For this review, take the finished solid that the model builds, in its own axes (mm). A direction names the side the tool comes from. Round coordinates to 2 decimals unless told otherwise and drop trailing zeros. Loops run counter-clockwise (first coordinate to the right, second up) from the corner with the lowest first, then second, coordinate; pieces in that order, holes last.
1. Consider section A-A on x = -49. State the section outline as (y, z) points (3 decimals).
2. Clearance check with flat-ended pins moving along their axes: pin 1 Ø3 at (y, z) = (-0.5, -6) entering from +X; pin 2 Ø8 at (x, z) = (-28, -1.5) entering from +Y (3 decimals); pin 3 Ø8 at (x, z) = (-22.5, 0.5) entering from -Y (3 decimals). State where each tip first meets the part, or that it passes through.
3. Draft analysis for pull direction X (two halves, no side actions). For faces 1 (the cylindrical face through (-14.31, 2.33, -0.52)), 2 (the cylindrical face through (-8, 3.1, -0.69)), 3 (the conical face through (-58.165, -1.259, 3.996)), 4 (the flat face through (-63.5, 0, 0)), state which applies: released by +X, released by -X, zero draft, split by the parting line, or undercut.
4. To check wall thickness, follow line 1 along X through (y, z) = (-5.75, -7.25); line 2 along Y through (x, z) = (-6.5, 0.5); line 3 along Z through (x, y) = (-23, 2). State the ranges of each line that lie inside material, in increasing order.
5. Tool access review of faces 5 (the cylindrical face through (-37.48, 3.1, -0.69)), 6 (the cylindrical face through (-61.935, 5.796, -7.559)): name each direction out of +Z, -Z, +X, -X, +Y, -Y from which nothing blocks a thin tool from reaching the whole face with its end or side.
from build123d import *


with BuildPart() as f1:
    # F0 (on Front) → F1 (revolve)
    with BuildSketch(Plane.XZ):
        with BuildLine():
            Line((-63.5, 9.525), (-63.5, 0))
            Line((-63.5, 0), (0, 0))
            ThreePointArc((0, 0), (-0.929936, 2.245064), (-3.175, 3.175))
            Line((-3.175, 3.175), (-12.7, 3.175))
            Line((-12.7, 3.175), (-12.7, 2.3876))
            Line((-12.7, 2.3876), (-15.875, 2.3876))
            Line((-15.875, 2.3876), (-17.238817, 3.175))
            Line((-17.238817, 3.175), (-57.161765, 3.175))
            ThreePointArc((-57.161765, 3.175), (-57.74161, 3.371831), (-58.081809, 3.880975))
            Line((-58.081809, 3.880975), (-59.404956, 8.819025))
            ThreePointArc((-59.404956, 8.819025), (-59.745155, 9.328169), (-60.325, 9.525))
            Line((-60.325, 9.525), (-63.5, 9.525))
        make_face()
    revolve(axis=Axis((-38.125068, 0, 0), (1, 0, 0)))


solid = f1.part
Resolved:
1. outline: circle Ø6.35 at (0, 0)
2. pin 1: stops at x = -58.25
2. pin 2: stops at y = 3.175
2. pin 3: stops at y = -3.175
3. face 1: undercut
3. face 2: zero draft
3. face 3: released by +X
3. face 4: released by -X
4. line 1: x = -63.5 to -59.66
4. line 2: y = -3.14 to 3.14
4. line 3: z = -2.47 to 2.47
5. face 5: +X
5. face 6: +X, -X
